Source: CAD feature listing. Evaluate the final solid. Frame: model axes, mm. Give positions to 0.01 mm unless a question says otherwise; leave off trailing zeros. Order: outer loops, then holes, each group sorted by start corner. A loop starts at its lowest first (then second) coordinate and runs counter-clockwise, first axis right, second up. Notation, with made-up numbers: M 86.5,87.5 L 124.5,87.5 A15 cw 124.5,109.5 Z; hole C 40,-39 d9. An arc over 180 degrees is marked long. Answer as a JSON object with one key per item and string values. Group by question number.
1. Pull-direction query (X, two-part tool) for faces 1 (the flat face through (39, 12.5, 6)), 2 (the cylindrical face through (18.526, 7.602, 6.162)), 3 (the cylindrical face through (76.908, 6.851, 6.162)), 4 (the flat face through (80, 6, 6)); classes: +X half, -X half, draft (parallel to the pull), parting line (faces both ways), or undercut.
2. Pin query (flat end, axial travel): P1, Ø5, axis at x = 75, y = 6.25, coming from the +Z side. Return the tip coordinate at first contact, or that it passes through.
3. Material intervals for L1, parallel to X at y = 6.25, z = 3.25; L2, parallel to Y at x = 60, z = 3.75; L3, parallel to X at y = 8, z = 9.5, sorted ascending. Write a range as [from, to].
4. Section query B-B (z = 4.5). Output: boundary loops of the cut face in (x, y), plus the area to 3 significant figures.
5. Section query C-C (y = 5.25). Output: boundary loops of the cut face in (x, z), plus the area to 3 significant figures.
6. Section query A-A (x = 20). Output: boundary loops of the cut face in (y, z).
from build123d import *

# Parameters (mm, degrees)
CYLINDER001_R     = 2
CYLINDER001_DEPTH = 13
CYLINDER002_R     = 2
CYLINDER002_DEPTH = 13
CYLINDER003_R     = 2
CYLINDER003_DEPTH = 13
CYLINDER_R        = 2
CYLINDER_DEPTH    = 13
BOX_W             = 80
BOX_H             = 12.5
BOX_DEPTH         = 12.5


with BuildPart() as cylinder001:
    # Cylinder001 → Cylinder001 (new body)
    with BuildSketch(Plane(origin=(20, 6.25, 0), x_dir=(1, 0, 0), z_dir=(0, 0, 1))):
        Circle(CYLINDER001_R)
    extrude(amount=CYLINDER001_DEPTH)


with BuildPart() as cylinder002:
    # Cylinder002 → Cylinder002 (new body)
    with BuildSketch(Plane(origin=(75, 6.25, 0), x_dir=(1, 0, 0), z_dir=(0, 0, 1))):
        Circle(CYLINDER002_R)
    extrude(amount=CYLINDER002_DEPTH)


with BuildPart() as cylinder003:
    # Cylinder003 → Cylinder003 (new body)
    with BuildSketch(Plane(origin=(60, 6.25, 0), x_dir=(1, 0, 0), z_dir=(0, 0, 1))):
        Circle(CYLINDER003_R)
    extrude(amount=CYLINDER003_DEPTH)


with BuildPart() as agujeroseje:
    # Cylinder → Cylinder (new body)
    with BuildSketch(Plane(origin=(5, 6.25, 0), x_dir=(1, 0, 0), z_dir=(0, 0, 1))):
        Circle(CYLINDER_R)
    extrude(amount=CYLINDER_DEPTH)

    # Compound: union Cylinder001, Cylinder002, Cylinder003
    add(cylinder001.part)
    add(cylinder002.part)
    add(cylinder003.part)


with BuildPart() as eje:
    # Box → Box (new body)
    with BuildSketch(Plane.XY):
        with Locations((40, 6.25)):
            Rectangle(BOX_W, BOX_H)
    extrude(amount=BOX_DEPTH)

    # Cut: cut AgujerosEje
    add(agujeroseje.part, mode=Mode.SUBTRACT)


solid = eje.part
Answer sheet:
{
 "1": {"face 1": "draft", "face 2": "undercut", "face 3": "undercut", "face 4": "+X half"},
 "2": {"P1": "z = 12.5"},
 "3": {"L1": "[0, 3], [7, 18], [22, 58], [62, 73], [77, 80]", "L2": "[0, 4.25], [8.25, 12.5]", "L3": "[0, 4.03], [5.97, 19.03], [20.97, 59.03], [60.97, 74.03], [75.97, 80]"},
 "4": {"outline": "M 0,0 L 80,0 L 80,12.5 L 0,12.5 Z; hole C 5,6.25 d4; hole C 20,6.25 d4; hole C 60,6.25 d4; hole C 75,6.25 d4", "area": "950 mm^2"},
 "5": {"outline": "M 0,0 L 3.27,0 L 3.27,12.5 L 0,12.5 Z; M 6.73,0 L 18.27,0 L 18.27,12.5 L 6.73,12.5 Z; M 21.73,0 L 58.27,0 L 58.27,12.5 L 21.73,12.5 Z; M 61.73,0 L 73.27,0 L 73.27,12.5 L 61.73,12.5 Z; M 76.73,0 L 80,0 L 80,12.5 L 76.73,12.5 Z", "area": "827 mm^2"},
 "6": {"outline": "M 0,0 L 4.25,0 L 4.25,12.5 L 0,12.5 Z; M 8.25,0 L 12.5,0 L 12.5,12.5 L 8.25,12.5 Z"}
}
